Geometry check sheet. Reference: the model listing, model coordinates, mm. A direction names the side the tool comes from. Give positions to 0.01 mm unless a question says otherwise; leave off trailing zeros. Loops run counter-clockwise (first coordinate to the right, second up) from the corner with the lowest first, then second, coordinate; pieces in that order, holes last. Notation, with made-up numbers: (79, 39) -> (88, 39) arc R30 ccw to (88, 62) -> close; hole circle Ø9 at (20.5, 43.25). An arc over 180 degrees is marked (long way). Answer as a JSON object with one key per item and string values.
from build123d import *

# Parameters (mm, degrees)
SKETCH1_W           = 28
SKETCH1_H           = 28
BOSS_EXTRUDE1_DEPTH = 20
CUT_EXTRUDE1_DEPTH  = 45.362146026
CUT_EXTRUDE2_REACH  = 43.952
SKETCH3_W           = 15
SKETCH3_H           = 26.880949604
CUT_EXTRUDE3_DEPTH  = 4
CUT_EXTRUDE4_DEPTH  = 4
SKETCH6_W           = 5.8
SKETCH6_H           = 1
BOSS_EXTRUDE2_DEPTH = 1
SKETCH7_W           = 1
SKETCH7_H           = 5.8
BOSS_EXTRUDE3_DEPTH = 1


with BuildPart() as part:
    # Sketch1 → Boss-Extrude1 (new body)
    with BuildSketch(Plane.XY):
        with Locations((14, 14)):
            Rectangle(SKETCH1_W, SKETCH1_H)
    extrude(amount=BOSS_EXTRUDE1_DEPTH)

    # Sketch2 → Cut-Extrude1 (cut, through all)
    with BuildSketch(Plane.XY.offset(20)):
        Polygon((5.5, 29.426142622), (5.5, 25.5), (25.5, 5.5), (30.244346823, 5.5), (30.244346823, 29.426142622), align=None)
    extrude(amount=-CUT_EXTRUDE1_DEPTH, mode=Mode.SUBTRACT)

    # Cut-Extrude2: up to this face of the body (flat: up to its plane)
    cut_extrude2_end = Plane(part.part.faces().sort_by_distance((28, 2.75, 10))[0])
    # Sketch3 → Cut-Extrude2 (cut, up to the picked face)
    with BuildSketch(Plane.ZY.offset(-4), mode=Mode.PRIVATE) as cut_extrude2_sk1:
        with Locations((10, 17.440474802)):
            Rectangle(SKETCH3_W, SKETCH3_H)
    cut_extrude2_tool1 = split(extrude(cut_extrude2_sk1.sketch, amount=-CUT_EXTRUDE2_REACH, mode=Mode.PRIVATE), bisect_by=cut_extrude2_end, keep=Keep.BOTH, mode=Mode.PRIVATE)
    add(cut_extrude2_tool1.solids().sort_by(Axis((4, 17.440475, 10), (1, 0, 0)))[0], mode=Mode.SUBTRACT)

    # Sketch4 → Cut-Extrude3 (cut)
    with BuildSketch(Plane(origin=(4, 0, 0), x_dir=(0, 0, -1), z_dir=(1, 0, 0))):
        with BuildLine():
            Line((-13, 19), (-13, 9))
            ThreePointArc((-13, 9), (-10, 6), (-7, 9))
            Line((-7, 9), (-7, 19))
            ThreePointArc((-7, 19), (-10, 22), (-13, 19))
        make_face()
    extrude(amount=-CUT_EXTRUDE3_DEPTH, mode=Mode.SUBTRACT)

    # Sketch5 → Cut-Extrude4 (cut)
    with BuildSketch(Plane(origin=(0, 4, 0), x_dir=(1, 0, 0), z_dir=(0, 1, 0))):
        with BuildLine():
            Line((19, -13), (9, -13))
            ThreePointArc((9, -13), (6, -10), (9, -7))
            Line((9, -7), (19, -7))
            ThreePointArc((19, -7), (22, -10), (19, -13))
        make_face()
    extrude(amount=-CUT_EXTRUDE4_DEPTH, mode=Mode.SUBTRACT)

    # Sketch6 → Boss-Extrude2 (add)
    with BuildSketch(Plane.ZY):
        with Locations((10, 26.5)):
            Rectangle(SKETCH6_W, SKETCH6_H)
    extrude(amount=BOSS_EXTRUDE2_DEPTH)

    # Sketch7 → Boss-Extrude3 (add)
    with BuildSketch(Plane.XZ):
        with Locations((26.5, 10)):
            Rectangle(SKETCH7_W, SKETCH7_H)
    extrude(amount=BOSS_EXTRUDE3_DEPTH)


solid = part.part
1) Section check B-B on z = 10. Record the cut outline in (x, y), plus the area to 3 significant figures.
Geometry check:
{"outline": "(-1, 26) -> (0, 26) -> (0, 22) -> (4, 22) -> (4, 28) -> (0, 28) -> (0, 27) -> (-1, 27) -> close; (0, 0) -> (6, 0) -> (6, 4) -> (4, 4) -> (4, 6) -> (0, 6) -> close; (22, 0) -> (26, 0) -> (26, -1) -> (27, -1) -> (27, 0) -> (28, 0) -> (28, 4) -> (22, 4) -> close", "area": "82.0 mm2"}
2) Material ranges on line 1 along Z through (x, y) = (1.75, 10.25); line 2 along Z through (x, y) = (12, 7.5); line 3 along Y through (x, z) = (9, 16), recorded low to high. Write a range as from..to.
Geometry check:
{"line 1": "z = 0..7, 13..20", "line 2": "z = 0..2.5, 17.5..20", "line 3": "y = 0..4"}
3) Section check C-C on y = 10.25. Record the cut outline in (x, z), plus the area to 3 significant figures.
Geometry check:
{"outline": "(0, 0) -> (20.75, 0) -> (20.75, 2.5) -> (4, 2.5) -> (4, 7) -> (0, 7) -> close; (0, 13) -> (4, 13) -> (4, 17.5) -> (20.75, 17.5) -> (20.75, 20) -> (0, 20) -> close", "area": "140 mm2"}
4) Tool access check on faces 4 (the face through (4, 16.2, 6.6)), 5 (the face through (26.5, -0.5, 12.9)), 6 (the face through (26.5, -0.5, 7.1)). Record the directions out of +Z, -Z, +X, -X, +Y, -Y that give a thin tool (end or side, any length) a straight path to the whole face; none if there is none.
Geometry check:
{"face 4": "+X, +Y", "face 5": "+Z, +X, -X, -Y", "face 6": "-Z, +X, -X, -Y"}
5) Depth check by flat-ended pin: P1, Ø6, axis at y = 19, z = 12, coming from the -X side; P2, Ø2, axis at x = 9.5, z = 10.5, coming from the +Y side; P3, Ø0.8, axis at y = 26.5, z = 18, coming from the +X side; P4, Ø10, axis at x = 24.5, z = 6, coming from the -Y side. Enter the tip coordinate at first touch or a pass-through.
Geometry check:
{"P1": "stops at x = 0", "P2": "passes through", "P3": "stops at x = 5.5", "P4": "stops at y = -1"}
6) Draft check along Y on faces 1 (the face through (-0.5, 26, 10)), 2 (the face through (15, 16, 19)), 3 (the face through (2, 6, 10)). Enter one of: pulls with the +Y half, pulls with the -Y half, needs draft (parallel to the pull), parting line crosses it, or undercut.
Geometry check:
{"face 1": "pulls with the -Y half", "face 2": "pulls with the +Y half", "face 3": "undercut"}
7) Section check D-D on x = 15. Record the cut outline in (y, z), plus the area to 3 significant figures.
Geometry check:
{"outline": "(0, 0) -> (16, 0) -> (16, 2.5) -> (4, 2.5) -> (4, 7) -> (0, 7) -> close; (0, 13) -> (4, 13) -> (4, 17.5) -> (16, 17.5) -> (16, 20) -> (0, 20) -> close", "area": "116 mm2"}
8) Section check A-A on x = 2. Record the cut outline in (y, z).
Geometry check:
{"outline": "(0, 0) -> (28, 0) -> (28, 20) -> (0, 20) -> close; hole (9, 7) -> (19, 7) arc R3 ccw to (19, 13) -> (9, 13) arc R3 ccw to start"}
